from build123d import *

# Parameters (mm, degrees)
CUT_EXTRUDE1_DEPTH = 0.83
CHAMFER2_SIZE      = 0.05


with BuildPart() as part:
    # Sketch1 → Revolve1 (revolve)
    with BuildSketch(Plane.XY):
        Polygon((-4.212732686, 1.5), (-5.462732686, 2.75), (-5.862732686, 2.75), (-5.862732686, 0), (4.137267314, 0), (4.137267314, 1.1), (3.737267314, 1.5), align=None)
    revolve(axis=Axis((48.184792793, 0, 0), (-1, 0, 0)))

    # Sketch2 → Cut-Extrude1 (cut)
    with BuildSketch(Plane.ZY.offset(5.862732686)):
        with BuildLine():
            ThreePointArc((1.16663108, 0.344585397), (1.212435565, 0.7), (0.881735248, 0.838039454))
            ThreePointArc((0.881735248, 0.838039454), (0.5125, 0.887676039), (0.284895833, 1.182624851))
            ThreePointArc((0.284895833, 1.182624851), (0, 1.4), (-0.284895833, 1.182624851))
            ThreePointArc((-0.284895833, 1.182624851), (-0.5125, 0.887676039), (-0.881735248, 0.838039454))
            ThreePointArc((-0.881735248, 0.838039454), (-1.212435565, 0.7), (-1.16663108, 0.344585397))
            ThreePointArc((-1.16663108, 0.344585397), (-1.025, 0), (-1.16663108, -0.344585397))
            ThreePointArc((-1.16663108, -0.344585397), (-1.212435565, -0.7), (-0.881735248, -0.838039454))
            ThreePointArc((-0.881735248, -0.838039454), (-0.5125, -0.887676039), (-0.284895833, -1.182624851))
            ThreePointArc((-0.284895833, -1.182624851), (0, -1.4), (0.284895833, -1.182624851))
            ThreePointArc((0.284895833, -1.182624851), (0.5125, -0.887676039), (0.881735248, -0.838039454))
            ThreePointArc((0.881735248, -0.838039454), (1.212435565, -0.7), (1.16663108, -0.344585397))
            ThreePointArc((1.16663108, -0.344585397), (1.025, 0), (1.16663108, 0.344585397))
        make_face()
    extrude(amount=-CUT_EXTRUDE1_DEPTH, mode=Mode.SUBTRACT)

    # Chamfer2
    chamfer2_edges = [part.edges().sort_by_distance(p)[0] for p in [
        (-5.862732686, 0.887676039, 0.5125),
        (-5.862732686, 0, 1.025),
        (-5.862732686, -0.887676039, 0.5125),
        (-5.862732686, -0.887676039, -0.5125),
        (-5.862732686, 0, -1.025),
        (-5.862732686, 0.887676039, -0.5125),
        (-5.862732686, 1.4, 0),
        (-5.862732686, 0.7, -1.212435565),
        (-5.862732686, -0.7, -1.212435565),
        (-5.862732686, -1.4, 0),
        (-5.862732686, -0.7, 1.212435565),
        (-5.862732686, 0.7, 1.212435565),
    ]]
    chamfer(chamfer2_edges, length=CHAMFER2_SIZE)


solid = part.part
Geometry: final body of the model. Coordinates: model frame, mm. A direction names the side the tool comes from. Give positions to 0.01 mm unless a question says otherwise; leave off trailing zeros. Write each loop counter-clockwise with the first axis right and the second up, starting at its lowest first coordinate (ties: lowest second). Pieces come first, ordered by that corner, then holes. Notation, with made-up numbers: M 11,23 L 64,23 A23 ccw 64,53 Z; hole C -2.75,-30 d3. An arc over 180 degrees is marked long. Answer in a Markdown table with one row per item. Add a question column.
(1) Reachability of faces 1 (the cylindrical face through (-0.29, -1.5, -0.07)), 2 (the flat face through (-5.863, 1.2, 0.6)) from +Z, -Z, +X, -X, +Y, -Y: full face, straight path, thin tool, end or side. Return the list, or none.
(2) Ray query, line 1 (Y direction, x = -3.5, z = 0); line 2 (X direction, y = 0.3, z = -0.95). Return the intervals inside material, ascending.
(3) Section B-B on x = 3. Return loops of the section in (y, z), and give its area (3 significant figures).
(4) Section A-A on z = 0. Return loops of the section in (x, y), and give its area (3 significant figures).
(5) Mould query, pull axis Z, two halves, no side actions, for faces 3 (the flat face through (-5.033, 0, 0)), 4 (the cylindrical face through (-5.666, -0.596, 2.685)), 5 (the flat face through (4.137, 0, 0)). Classes: +Z half, -Z half, draft (parallel to the pull), parting line (faces both ways), or undercut.
(6) Section C-C on y = 0. Return loops of the section in (x, z) (3 decimals).
(7) First-contact query: pin 1 (3 mm diameter, centred on x = -3, y = -1.5, fed in from +Z); pin 2 (3 mm diameter, centred on x = -3, z = 1.5, fed in from +Y); pin 3 (1 mm diameter, centred on x = 1.5, y = -0.5, fed in from -Z). Flat tips, straight axial feed; report the tip coordinate or a pass-through.
Result set:
| question | item | result |
|---|---|---|
| 1 | face 1 | +X |
| 1 | face 2 | +Z, -Z, -X, +Y, -Y |
| 2 | line 1 | y = -1.5 to 1.5 |
| 2 | line 2 | x = -5.03 to 4.14 |
| 3 | outline | C 0,0 d3 |
| 3 | area | 7.07 mm^2 |
| 4 | outline | M -5.86,-2.75 L -5.46,-2.75 L -4.21,-1.5 L 3.74,-1.5 L 4.14,-1.1 L 4.14,1.1 L 3.74,1.5 L -4.21,1.5 L -5.46,2.75 L -5.86,2.75 L -5.86,1.45 L -5.81,1.4 L -5.03,1.4 L -5.03,-1.4 L -5.81,-1.4 L -5.86,-1.45 Z |
| 4 | area | 30.1 mm^2 |
| 5 | face 3 | undercut |
| 5 | face 4 | parting line |
| 5 | face 5 | draft |
| 6 | outline | M -5.863,-2.75 L -5.463,-2.75 L -4.213,-1.5 L 3.737,-1.5 L 4.137,-1.1 L 4.137,1.1 L 3.737,1.5 L -4.213,1.5 L -5.463,2.75 L -5.863,2.75 L -5.863,1.075 L -5.813,1.025 L -5.033,1.025 L -5.033,-1.025 L -5.813,-1.025 L -5.863,-1.075 Z |
| 7 | pin 1 | stops at z = 1.5 |
| 7 | pin 2 | stops at y = 1.5 |
| 7 | pin 3 | stops at z = -1.5 |
